Read the model definition and answer for the solid it produces. Units are mm, in the model's axes. A direction names the side the tool comes from. Give positions to 0.01 mm unless a question says otherwise; leave off trailing zeros. Write each loop counter-clockwise with the first axis right and the second up, starting at its lowest first coordinate (ties: lowest second). Pieces come first, ordered by that corner, then holes. Notation, with made-up numbers: (28, -38) -> (51, -38) arc R10 cw to (51, -24) -> close; hole circle Ø2 at (73.5, 34.25). An arc over 180 degrees is marked (long way). Answer as CSV lines item,"result". Start each with the question number.
1. The part is cut by section C-C, the plane y = 0. Determine the outline of the cut face in (x, z).
2. Given pin 1 (12 mm diameter, centred on x = -50.5, y = 6, fed in from -Z); pin 2 (4.5 mm diameter, centred on x = -56.5, z = 71.5, fed in from +Y); pin 3 (5 mm diameter, centred on y = 50.5, z = 39, fed in from +X); pin 4 (3 mm diameter, centred on x = -20.5, z = 35.5, fed in from +Y), each flat-ended and moving along its own axis, determine where each tip first touches the part or whether it passes through.
3. The part is cut by section A-A, the plane x = -56.5. Determine the outline of the cut face in (y, z).
4. The part is cut by section B-B, the plane z = 71.5. Determine the outline of the cut face in (x, y), and give its area (3 significant figures).
5. For a pull along X with two mould halves and no side action, classify faces 3 (the cylindrical face through (-68, 69, 39)), 4 (the cylindrical face through (-39.41, 67.46, 67.44)), 5 (the cylindrical face through (-54.883, 67.465, 34.83)), 6 (the flat face through (-33, -70, 39)) as pulls with the +X half, pulls with the -X half, needs draft (parallel to the pull), parting line crosses it, or undercut.
6. Find the intervals of material crossed by line 1 (Z direction, x = -20.5, y = 68.8); line 2 (Y direction, x = -47, z = 61); line 3 (Z direction, x = -38.5, y = -67.75), in increasing order.
7. The part is cut by section D-D, the plane z = 60.5. Determine the outline of the cut face in (x, y), and give its area (3 significant figures).
8. A tool of negligible diameter and unlimited length cuts with its end or side. For faces 1 (the cylindrical face through (-21.89, -67.54, 34.44)), 2 (the flat face through (-65, -1, 37)), from which of +Z, -Z, +X, -X, +Y, -Y can it reach the whole face along a straight path? Write none if from no direction.
from build123d import *

# Parameters (mm, degrees)
PAD_DEPTH       = 80
POCKET_DEPTH    = 75
SKETCH002_R     = 7
SKETCH002_R_2   = 1.75
POCKET001_DEPTH = 140


with BuildPart() as part:
    # Sketch → Pad (new body)
    with BuildSketch(Plane.XY):
        with BuildLine():
            Line((0, 70), (-65, 70))
            ThreePointArc((-65, 70), (-68.535534, 68.535534), (-70, 65))
            Line((-70, 65), (-70, -65))
            ThreePointArc((-70, -65), (-68.535534, -68.535534), (-65, -70))
            Line((-65, -70), (0, -70))
            ThreePointArc((0, -70), (70, 0), (0, 70))
        make_face()
    extrude(amount=PAD_DEPTH)

    # Sketch001 (on Face7 of Pad) → Pocket (cut)
    with BuildSketch(Plane(origin=(0, 0, 0), x_dir=(1, 0, 0), z_dir=(0, 0, -1))):
        with BuildLine():
            ThreePointArc((0, -65), (65.000059, 0), (0, 65))
            Line((0, 65), (-60, 65))
            ThreePointArc((-60, 65), (-63.535534, 63.535534), (-65, 60))
            Line((-65, 60), (-65, -60))
            ThreePointArc((-65, -60), (-63.535534, -63.535534), (-60, -65))
            Line((-60, -65), (0, -65))
        make_face()
    extrude(amount=-POCKET_DEPTH, mode=Mode.SUBTRACT)

    # Sketch002 (on Face6 of Pocket) → Pocket001 (cut)
    with BuildSketch(Plane.XZ.offset(70)):
        with Locations((-38.5, 60.5)):
            Circle(SKETCH002_R)
        with Locations((-56.5, 71.5)):
            Circle(SKETCH002_R_2)
        with Locations((-56.5, 35.5)):
            Circle(SKETCH002_R_2)
        with Locations((-20.5, 71.5)):
            Circle(SKETCH002_R_2)
        with Locations((-20.5, 35.5)):
            Circle(SKETCH002_R_2)
    extrude(amount=-POCKET001_DEPTH, mode=Mode.SUBTRACT)


solid = part.part
Results found:
1,outline,"(-70, 0) -> (-65, 0) -> (-65, 75) -> (65, 75) -> (65, 0) -> (70, 0) -> (70, 80) -> (-70, 80) -> close"
2,pin 1,"stops at z = 75"
2,pin 2,"stops at y = 70"
2,pin 3,"stops at x = 50.95"
2,pin 4,"passes through"
3,outline,"(-70, 0) -> (-65, 0) -> (-65, 33.75) -> (-70, 33.75) -> close; (-70, 37.25) -> (-65, 37.25) -> (-65, 69.75) -> (-70, 69.75) -> close; (-70, 73.25) -> (-65, 73.25) -> (-65, 75) -> (65, 75) -> (65, 73.25) -> (70, 73.25) -> (70, 80) -> (-70, 80) -> close; (65, 0) -> (70, 0) -> (70, 33.75) -> (65, 33.75) -> close; (65, 37.25) -> (70, 37.25) -> (70, 69.75) -> (65, 69.75) -> close"
4,outline,"(-70, -65) arc R5 ccw to (-65, -70) -> (-58.25, -70) -> (-58.25, -65) -> (-60, -65) arc R5 cw to (-65, -60) -> (-65, 60) arc R5 cw to (-60, 65) -> (-58.25, 65) -> (-58.25, 70) -> (-65, 70) arc R5 ccw to (-70, 65) -> close; (-54.75, -70) -> (-22.25, -70) -> (-22.25, -65) -> (-54.75, -65) -> close; (-54.75, 65) -> (-22.25, 65) -> (-22.25, 70) -> (-54.75, 70) -> close; (-18.75, -70) -> (0, -70) arc R70 ccw to (0, 70) -> (-18.75, 70) -> (-18.75, 65) -> (0, 65) arc R65 cw to (0, -65) -> (-18.75, -65) -> close"
4,area,"2,340 mm²"
5,face 3,"pulls with the -X half"
5,face 4,"undercut"
5,face 5,"undercut"
5,face 6,"needs draft"
6,line 1,"z = 0 to 33.75, 37.25 to 69.75, 73.25 to 80"
6,line 2,"y = -70 to -65, 65 to 70"
6,line 3,"z = 0 to 53.5, 67.5 to 80"
7,outline,"(-70, -65) arc R5 ccw to (-65, -70) -> (-45.5, -70) -> (-45.5, -65) -> (-60, -65) arc R5 cw to (-65, -60) -> (-65, 60) arc R5 cw to (-60, 65) -> (-45.5, 65) -> (-45.5, 70) -> (-65, 70) arc R5 ccw to (-70, 65) -> close; (-31.5, -70) -> (0, -70) arc R70 ccw to (0, 70) -> (-31.5, 70) -> (-31.5, 65) -> (0, 65) arc R65 cw to (0, -65) -> (-31.5, -65) -> close"
7,area,"2,270 mm²"
8,face 1,"+Y, -Y"
8,face 2,"-Z"
